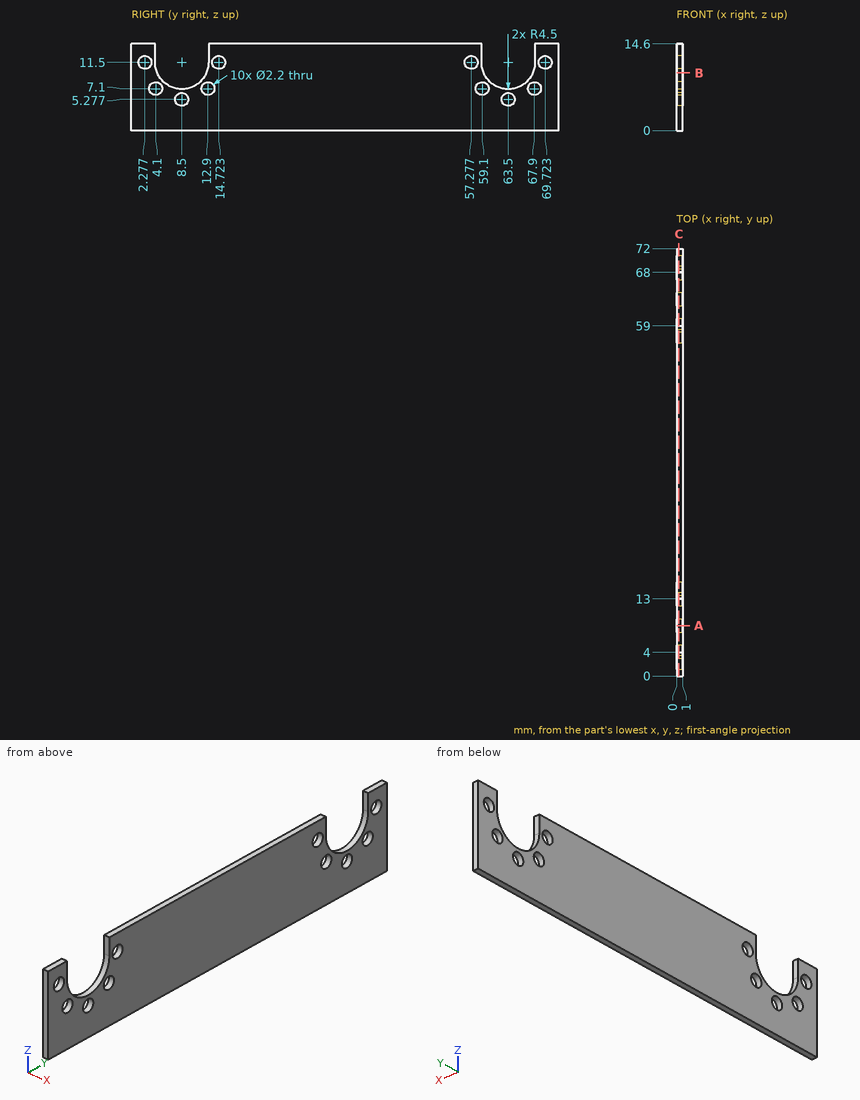
Check sheet for the drawn part. Datum: minimum x, y, z corner. Units: mm. Coordinates: 2 decimals unless noted, no trailing zeros. Order: outer loops, then holes, each group sorted by start corner. A loop starts at its lowest first (then second) coordinate and runs counter-clockwise, first axis right, second up. Notation, with made-up numbers: M 23.25,8 L 70.25,8 A14 ccw 70.25,33 Z; hole C -4.5,41 d7. An arc over 180 degrees is marked long. One line per question, with ' | ' between items. Start each with the question number.
Item 1: Material ranges on L1, parallel to Y at x = 0.75, z = 13; L2, parallel to Z at x = 0.7, y = 8.5; L3, parallel to Y at x = 0.95, z = 5.75 (1 decimal), recorded low to high. Write a range as [from, to].
Item 2: Gauge pin test, flat end, axial feed: pin 1 (1.8 mm diameter, centred on y = 8.5, z = 5.28, fed in from -X). Record the tip position at first contact, or that the pin passes through.
Item 3: Cross-section at A-A on y = 8.5. Enter the section's corners in (x, z).
Item 4: Cross-section at B-B on z = 9.75. Enter the section's corners in (x, y) (1 decimal).
Item 5: Cross-section at C-C on x = 0.35. State how many separate pieces and enclosed holes the cut face has, then the cut area to 3 significant figures.
Findings:
1) L1: y = [0, 4], [13, 59], [68, 72] | L2: z = [0, 4.18], [6.38, 7] | L3: y = [0, 7.5], [9.5, 62.5], [64.5, 72]
2) pin 1: passes through
3) outline: M 0,0 L 1,0 L 1,4.18 L 0,4.18 Z; M 0,6.38 L 1,6.38 L 1,7 L 0,7 Z
4) outline: M 0,0 L 1,0 L 1,4.4 L 0,4.4 Z; M 0,12.6 L 1,12.6 L 1,59.4 L 0,59.4 Z; M 0,67.6 L 1,67.6 L 1,72 L 0,72 Z
5) separate pieces: 1 | enclosed holes: 10 | area: 894 mm²
